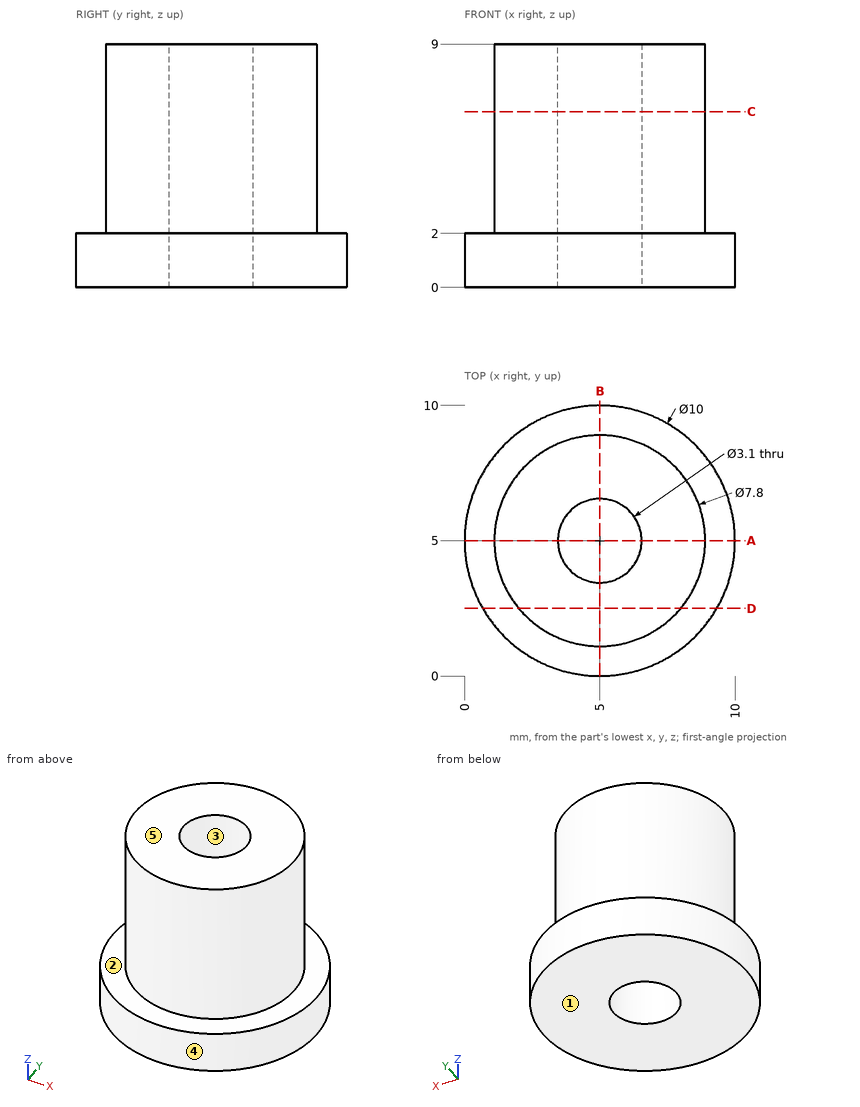
Study the drawing (mm; zero at the part's minimum x, y, z) and answer. A direction names the side the tool comes from. Give positions to 0.01 mm unless a question says otherwise; leave off trailing zeros. Order: outer loops, then holes, each group sorted by start corner. A loop starts at its lowest first (then second) coordinate and runs counter-clockwise, first axis right, second up. Notation, with made-up numbers: (14.25, 27) - (71.25, 27) arc R9 ccw to (71.25, 39) - close; hole circle Ø11 at (-28.5, -6.5). An arc over 180 degrees is marked (long way). Answer as CSV lines item,"result". Start each with the question number.
Q1. For the marked faces 1 and 2, determine the directions among +Z, -Z, +X, -X, +Y, -Y from which every point of the face is accessible in a straight line to the end or side of a thin tool.
Q2. The part is cut by section D-D (y = 2.5). Write down the section's boundary in (x, z), then the cut area to 3 significant figures.
Q3. Given pin 1 Ø5 at (y, z) = (6, 5.5) entering from -X; pin 2 Ø2 at (y, z) = (8, 2.5) entering from +X; pin 3 Ø1 at (y, z) = (7, 1.5) entering from +X; pin 4 Ø6 at (x, y) = (9, 7.5) entering from -Z, each flat-ended and moving along its own axis, determine where each tip first touches the part or whether it passes through.
Q4. The part is cut by section A-A (y = 5). Write down the section's boundary in (x, z).
Q5. The mould has two halves that part along X. Classify the marked faces 3, 4 and 5: +X half, -X half, draft (parallel to the pull), parting line (faces both ways), or undercut.
Q6. The part is cut by section C-C (z = 6.5). Write down the section's boundary in (x, y), then the cut area to 3 significant figures.
Q7. Find the intervals of material crossed by L1, parallel to Y at x = 5, z = 3.5; L2, parallel to Z at x = 8.5, y = 2.75; L3, parallel to Y at x = 5.5, z = 1.25, in increasing order. Write a range as [from, to].
Check result:
1,face 1,"-Z, +X, -X, +Y, -Y"
1,face 2,"+Z"
2,outline,"(0.67, 0) - (9.33, 0) - (9.33, 2) - (7.99, 2) - (7.99, 9) - (2.01, 9) - (2.01, 2) - (0.67, 2) - close"
2,area,"59.2 mm²"
3,pin 1,"stops at x = 1.1"
3,pin 2,"stops at x = 9.52"
3,pin 3,"stops at x = 9.77"
3,pin 4,"stops at z = 0"
4,outline,"(0, 0) - (3.45, 0) - (3.45, 9) - (1.1, 9) - (1.1, 2) - (0, 2) - close; (6.55, 0) - (10, 0) - (10, 2) - (8.9, 2) - (8.9, 9) - (6.55, 9) - close"
5,face 3,"undercut"
5,face 4,"parting line"
5,face 5,"draft"
6,outline,"circle Ø7.8 at (5, 5); hole circle Ø3.1 at (5, 5)"
6,area,"40.2 mm²"
7,L1,"y = [1.1, 3.45], [6.55, 8.9]"
7,L2,"z = [0, 2]"
7,L3,"y = [0.03, 3.53], [6.47, 9.97]"
